Can you work these out from the model? Positions are in its coordinate system, mm. A direction names the side the tool comes from. Give positions to 0.01 mm unless a question says otherwise; leave off trailing zeros. Loops run counter-clockwise (first coordinate to the right, second up) from the corner with the lowest first, then second, coordinate; pieces in that order, holes last.
from build123d import *

# Parameters (mm, degrees)
BASE_FLANGE1_DEPTH = 101.6
SKETCH7_R          = 2.4892
CUT_EXTRUDE1_DEPTH = 125.434078933
SKETCH8_R          = 2.4892
CUT_EXTRUDE2_DEPTH = 125.434078933
FILLET1_R          = 6.35


# Sheet-metal steps are written as plain solids
with BuildPart() as part:
    # Sketch2 → Base-Flange1 (new body)
    with BuildSketch(Plane(origin=(0, 0, 0), x_dir=(1, 0, 0), z_dir=(0, 1, 0))):
        with BuildLine():
            Line((0, -50.8), (0, -4.191))
            ThreePointArc((0, -4.191), (1.22751548, -1.22751548), (4.191, 0))
            Line((4.191, 0), (50.8, 0))
            Line((50.8, 0), (50.8, -3.429))
            Line((50.8, -3.429), (4.191, -3.429))
            ThreePointArc((4.191, -3.429), (3.652184633, -3.652184633), (3.429, -4.191))
            Line((3.429, -4.191), (3.429, -50.8))
            Line((3.429, -50.8), (0, -50.8))
        make_face()
    extrude(amount=BASE_FLANGE1_DEPTH)

    # Sketch7 → Cut-Extrude1 (cut, through all)
    with BuildSketch(Plane.ZY):
        with Locations((38.1, 88.9)):
            Circle(SKETCH7_R)
        with Locations((12.7, 88.9)):
            Circle(SKETCH7_R)
        with Locations((12.7, 63.5)):
            Circle(SKETCH7_R)
        with Locations((12.7, 38.1)):
            Circle(SKETCH7_R)
        with Locations((12.7, 12.7)):
            Circle(SKETCH7_R)
        with Locations((38.1, 63.5)):
            Circle(SKETCH7_R)
        with Locations((38.1, 38.1)):
            Circle(SKETCH7_R)
        with Locations((38.1, 12.7)):
            Circle(SKETCH7_R)
    extrude(amount=-CUT_EXTRUDE1_DEPTH, mode=Mode.SUBTRACT)

    # Sketch8 → Cut-Extrude2 (cut, through all)
    with BuildSketch(Plane(origin=(0, 0, 0), x_dir=(-1, 0, 0), z_dir=(0, 0, -1))):
        with Locations((-38.1, 88.9)):
            Circle(SKETCH8_R)
        with Locations((-12.7, 88.9)):
            Circle(SKETCH8_R)
        with Locations((-12.7, 63.5)):
            Circle(SKETCH8_R)
        with Locations((-12.7, 38.1)):
            Circle(SKETCH8_R)
        with Locations((-12.7, 12.7)):
            Circle(SKETCH8_R)
        with Locations((-38.1, 63.5)):
            Circle(SKETCH8_R)
        with Locations((-38.1, 38.1)):
            Circle(SKETCH8_R)
        with Locations((-38.1, 12.7)):
            Circle(SKETCH8_R)
    extrude(amount=-CUT_EXTRUDE2_DEPTH, mode=Mode.SUBTRACT)

    # Fillet1
    fillet1_edges = [part.edges().sort_by_distance(p)[0] for p in [
        (1.7145, 101.6, 50.8),
        (1.7145, 0, 50.8),
        (50.8, 101.6, 1.7145),
        (50.8, 0, 1.7145),
    ]]
    fillet(fillet1_edges, radius=FILLET1_R)


solid = part.part
(1) Suppose I cut it at B-B on z = 38.1. List the corners of the cut face in (x, y) for me.
Returned:
outline: (0, 0) - (3.43, 0) - (3.43, 10.21) - (0, 10.21) - close; (0, 15.19) - (3.43, 15.19) - (3.43, 35.61) - (0, 35.61) - close; (0, 40.59) - (3.43, 40.59) - (3.43, 61.01) - (0, 61.01) - close; (0, 65.99) - (3.43, 65.99) - (3.43, 86.41) - (0, 86.41) - close; (0, 91.39) - (3.43, 91.39) - (3.43, 101.6) - (0, 101.6) - close
(2) Suppose I cut it at D-D on y = 26. List the corners of the cut face in (x, z) for me, plus the area to 3 significant figures.
Returned:
outline: (0, 4.19) arc R4.19 ccw to (4.19, 0) - (50.8, 0) - (50.8, 3.43) - (4.19, 3.43) arc R0.76 cw to (3.43, 4.19) - (3.43, 50.8) - (0, 50.8) - close
area: 333 mm2
(3) Will these pins go through, and if not, where does the flat tip stop? P1, Ø4, axis at y = 88.9, z = 38.1, coming from the -X side; P2, Ø1, axis at x = 33, y = 86, coming from the +Z side; P3, Ø4, axis at y = 27.5, z = 45.5, coming from the +X side.
Returned:
P1: passes through
P2: stops at z = 3.43
P3: stops at x = 3.43
(4) Thinking about a two-plate mould opening in X: for faces 1 (the cylindrical face through (1.195, 50.089, 1.26)), 2 (the cylindrical face through (1.69, 15.17, 12.38)), 3 (the cylindrical face through (36.76, 91, 1.69)), which applies, pulls with the +X half, pulls with the -X half, needs draft (parallel to the pull), parting line crosses it, or undercut?
Returned:
face 1: pulls with the -X half
face 2: needs draft
face 3: undercut
(5) Suppose I cut it at A-A on x = 38.1. List the corners of the cut face in (y, z) for me.
Returned:
outline: (0, 0) - (10.21, 0) - (10.21, 3.43) - (0, 3.43) - close; (15.19, 0) - (35.61, 0) - (35.61, 3.43) - (15.19, 3.43) - close; (40.59, 0) - (61.01, 0) - (61.01, 3.43) - (40.59, 3.43) - close; (65.99, 0) - (86.41, 0) - (86.41, 3.43) - (65.99, 3.43) - close; (91.39, 0) - (101.6, 0) - (101.6, 3.43) - (91.39, 3.43) - close
(6) Please list where these lines run through material, in increasing order: probe 1 along Y at (x, z) = (12.7, 2.4); probe 2 along Z at (x, y) = (1, 38); probe 3 along Y at (x, z) = (1, 12).
Returned:
probe 1: y = 0 to 10.21, 15.19 to 35.61, 40.59 to 61.01, 65.99 to 86.41, 91.39 to 101.6
probe 2: z = 1.47 to 10.21, 15.19 to 35.61, 40.59 to 50.8
probe 3: y = 0 to 10.31, 15.09 to 35.71, 40.49 to 61.11, 65.89 to 86.51, 91.29 to 101.6
(7) Which directions (+Z, -Z, +X, -X, +Y, -Y) give clear straight access to the entire face, cutting with the end or side of a thin tool? Please do faces 4 (the cylindrical face through (38.64, 35.67, 1.69)), 5 (the flat face through (3.429, 50, 27)).
Returned:
face 4: +Z, -Z
face 5: +Z, +X, +Y, -Y
(8) Suppose I cut it at C-C on y = 88.9. List the corners of the cut face in (x, z) for me.
Returned:
outline: (0, 4.19) arc R4.19 ccw to (4.19, 0) - (10.21, 0) - (10.21, 3.43) - (4.19, 3.43) arc R0.76 cw to (3.43, 4.19) - (3.43, 10.21) - (0, 10.21) - close; (0, 15.19) - (3.43, 15.19) - (3.43, 35.61) - (0, 35.61) - close; (0, 40.59) - (3.43, 40.59) - (3.43, 50.8) - (0, 50.8) - close; (15.19, 0) - (35.61, 0) - (35.61, 3.43) - (15.19, 3.43) - close; (40.59, 0) - (50.8, 0) - (50.8, 3.43) - (40.59, 3.43) - close
